Source: CAD feature listing. Evaluate the final solid. Frame: model axes, mm. Face numbers are marked on the shaded views. A direction names the side the tool comes from. Coordinates: 2 decimals unless noted, no trailing zeros. Write each loop counter-clockwise with the first axis right and the second up, starting at its lowest first coordinate (ties: lowest second). Pieces come first, ordered by that corner, then holes. Notation, with made-up numbers: (11.5, 14.25) -> (18.5, 14.25) arc R16 ccw to (18.5, 38.25) -> close; hole circle Ø7 at (76, 12.25). An arc over 180 degrees is marked (long way). One line per item, written item: value. Start each with the question number.
1. Section query A-A, the plane x = -12.7. State how many separate pieces and enclosed holes the cut face has, and give its area (3 significant figures).
2. First-contact query: P1, Ø4, axis at x = -20.64, y = 38.1, coming from the -Z side; P2, Ø7.5, axis at x = -44.45, y = 38.1, coming from the -Z side; P3, Ø12.5, axis at x = -21.5, z = -4, coming from the +Y side; P4, Ø8, axis at y = 25, z = -43.5, coming from the -X side. Flat tips, straight axial feed; report the tip coordinate or a pass-through.
3. Mould query, pull axis Z, two halves, no side actions, for the marked faces 5, 6 and 7. Classes: released by +Z, released by -Z, zero draft, split by the parting line, or undercut.
4. Section query B-B, the plane y = -24. Output: boundary loops of the cut face in (x, z), and give its area (3 significant figures).
5. Line query: line 1 (Y direction, x = -44.45, z = -15.25) (3 decimals); line 2 (Y direction, x = -12, z = -50); line 3 (Y direction, x = -8.5, z = -30). Output: solid intervals per line, ascending.
6. Access query for the marked faces 1, 2, 3 and 4. Directions: +Z, -Z, +X, -X, +Y, -Y. A direction counts if a zero-diameter tool reaches every point of the face in a straight line with its end or side. Return the directions, or none.
7. Section query D-D, the plane x = 5.5. Output: boundary loops of the cut face in (y, z), and give its area (3 significant figures).
8. Section query C-C, the plane y = 10.5. Output: boundary loops of the cut face in (x, z), and give its area (3 significant figures).
Autodesk Inventor part; units mm, degrees
ref_plane "Work Plane1" through (0, 0, -31.75) normal (0, 0, 1) x (1, 0, 0)
ref_plane "Work Plane2" through (0, 31.75, -63.5) normal (0, -1, 0) x (1, 0, 0)
ref_plane "YZ Plane" through (0, 0, 0) normal (1, 0, 0) x (0, 1, 0)
sketch "Sketch1" plane through (0, 0, 0) normal (0, 0, 1) x (1, 0, 0)
  arc A0 (-50.8, 31.75) -> (-50.8, -31.75) centre (-50.8, 0) ccw
  line L0 (-50.8, 31.75) -> (0, 31.75)
  line L1 (0, -31.75) -> (-50.8, -31.75)
  arc A1 (0, -31.75) -> (0, 31.75) centre (0, 0) ccw
extrude "Extrusion1" add sketch "Sketch1" against normal blind 63.5
ref_plane "Work Plane1" through (0, 0, -31.75) normal (0, 0, 1) x (1, 0, 0)
sketch "Sketch2" plane through (0, 0, -31.75) normal (0, 0, 1) x (1, 0, 0)
  arc A0 (-50.8, 31.75) -> (-50.8, -31.75) centre (-50.8, 0) ccw
  line L0 (-50.8, 31.75) -> (0, 31.75)
  arc A1 (0, -31.75) -> (0, 31.75) centre (0, 0) ccw
  line L1 (0, -31.75) -> (-50.8, -31.75)
  arc A2 (-50.8, 28.1437) -> (-50.8, -28.1437) centre (-50.8, 0) ccw
  line L2 (-50.8, 28.1437) -> (0, 28.1437)
  arc A3 (0, -28.1437) -> (0, 28.1437) centre (0, 0) ccw
  line L3 (0, -28.1437) -> (-50.8, -28.1437)
extrude "Extrusion2" cut sketch "Sketch2" along normal mid plane 55.88 contours L2 A3 L3 A2
sketch "Sketch3" plane through (0, 0, 0) normal (0, 0, 1) x (1, 0, 0)
  circle A0 centre (0, 0) radius 31.75
  line L0 (0, 31.75) -> (19.0425, -25.4056)
  dimension "d7" = 63.5
extrude "Extrusion3" cut sketch "Sketch3" against normal blind 63.5 contours A0 L0 picked at (8.7025, 12.4328)
sketch "Sketch4" plane through (-50.8, 31.75, 0) normal (0, 1, 0) x (1, 0, 0)
  line L0 (50.8, 0) -> (0, 0)
  line L1 (50.8, 0) -> (50.8, 63.5)
  line L2 (0, 63.5) -> (50.8, 63.5)
  line L3 (0, 0) -> (0, 63.5)
  line L4 (0, 31.75) -> (50.8, 31.75)
  line L5 (0, 0) -> (0, 63.5)
  line L6 (50.8, 0) -> (50.8, 63.5)
  line L7 (0, 11.43) -> (50.8, 11.43)
  line L8 (50.8, 11.43) -> (50.8, 52.07)
  line L9 (50.8, 52.07) -> (0, 52.07)
  line L10 (0, 52.07) -> (0, 11.43)
  line L11 (0, 19.3675) -> (50.8, 19.3675)
  line L12 (0, 44.1325) -> (50.8, 44.1325)
  dimension "d10" = 31.75
  dimension "d11" = 20.32
  dimension "d12" = 40.64
  dimension "d13" = 7.9375
  dimension "d14" = 7.9375
extrude "Extrusion4" add sketch "Sketch4" along normal blind 12.7 contours L7 L3 L11 L1 | L12 L3 L9 L1
sketch "Sketch5" plane through (-50.8, 31.75, -11.43) normal (0, 0, 1) x (1, 0, 0)
  line L0 (50.8, 0) -> (0, 0)
  line L1 (50.8, 0) -> (50.8, 12.7)
  line L2 (0, 12.7) -> (50.8, 12.7)
  line L3 (0, 0) -> (0, 12.7)
  circle A0 centre (6.35, 6.35) radius 6.35
  circle A1 centre (44.45, 6.35) radius 6.35
  line L4 (6.35, 12.7) -> (44.45, 12.7)
  line L5 (44.45, 0) -> (6.35, 0)
  line L6 (6.35, 6.35) -> (0, 6.35)
  line L7 (44.45, 6.35) -> (50.8, 6.35)
  point P0 (50.8, -31.75)
extrude "Extrusion5" cut sketch "Sketch5" against normal blind 63.5 contours A1 L2 L1 | L3 L2 A0
sketch "Sketch6" plane through (-50.8, 31.75, -11.43) normal (0, 0, 1) x (1, 0, 0)
  arc A0 (6.35, 12.7) -> (0, 6.35) centre (6.35, 6.35) ccw
  line L0 (0, 0) -> (0, 6.35)
  line L1 (50.8, 0) -> (0, 0)
  line L2 (50.8, 0) -> (50.8, 6.35)
  arc A1 (50.8, 6.35) -> (44.45, 12.7) centre (44.45, 6.35) ccw
  line L3 (6.35, 12.7) -> (44.45, 12.7)
  circle A2 centre (6.35, 6.35) radius 3.175
  line L4 (6.35, 6.35) -> (44.45, 6.35)
  circle A3 centre (14.2875, 6.35) radius 3.175
  circle A4 centre (22.225, 6.35) radius 3.175
  circle A5 centre (30.1625, 6.35) radius 3.175
  circle A6 centre (38.1, 6.35) radius 3.175
  point P0 (50.8, -31.75)
  dimension "d22" = 7.9375
  dimension "d31" = 6.35
extrude "Extrusion6" cut sketch "Sketch6" against normal blind 63.5 contours A2 | A6 L4 | L4 A6 | A5 L4 | L4 A5 | A4 L4 | L4 A4 | A3 L4 | L4 A3
ref_plane "Work Plane2" through (0, 31.75, -63.5) normal (0, -1, 0) x (1, 0, 0)
sketch "Sketch8" plane through (0, 31.75, -63.5) normal (0, -1, 0) x (1, 0, 0)
  line L0 (-50.8, 63.5) -> (-50.8, 63.5)
  line L1 (-50.8, 63.5) -> (-50.8, 52.07)
  line L2 (-50.8, 52.07) -> (-50.8, 44.1325)
  line L3 (-50.8, 44.1325) -> (-50.8, 19.3675)
  line L4 (-50.8, 19.3675) -> (-50.8, 11.43)
  line L5 (-50.8, 11.43) -> (-50.8, 0)
  line L6 (-50.8, 0) -> (-50.8, 0)
  line L7 (-50.8, 63.5) -> (-50.8, 0)
  line L8 (-50.8, 63.5) -> (-82.55, 63.5)
  line L9 (-82.55, 63.5) -> (-82.55, 0)
  line L10 (-82.55, 0) -> (-50.8, 0)
  line L11 (-50.8, 59.69) -> (-78.9437, 59.69)
  line L12 (-54.4877, 59.69) -> (-50.8, 59.69)
  line L13 (-78.9437, 3.81) -> (-78.9437, 59.69)
  line L14 (-50.8, 59.69) -> (-82.55, 59.69)
  line L15 (-78.9437, 59.69) -> (-78.9437, 3.81)
  line L16 (-82.55, 3.81) -> (-50.8, 3.81)
  line L17 (-50.8, 3.81) -> (-50.8, 59.69)
  line L18 (-82.55, 59.69) -> (-82.55, 3.81)
  line L19 (-50.8, 63.5) -> (-82.55, 63.5)
  line L20 (-82.55, 63.5) -> (-82.55, 59.69)
  line L21 (-82.55, 59.69) -> (-50.8, 59.69)
  line L22 (-50.8, 59.69) -> (-50.8, 63.5)
  line L23 (-78.9437, 59.69) -> (-50.8, 59.69)
  line L24 (-50.8, 59.69) -> (-50.8, 3.81)
  line L25 (-50.8, 3.81) -> (-78.9437, 3.81)
  line L26 (-78.9437, 3.81) -> (-78.9437, 59.69)
  line L27 (-82.55, 3.81) -> (-50.8, 3.81)
  line L28 (-50.8, 3.81) -> (-50.8, 0)
  line L29 (-50.8, 0) -> (-82.55, 0)
  line L30 (-82.55, 0) -> (-82.55, 3.81)
  point P0 (0, 63.5)
extrude "Extrusion7" cut sketch "Sketch8" along normal blind 31.75 contours L1 L2 L3 L4 L5 L16 L13 L11 | L14 L13 L16 L9
properties part number "Scoop_001"
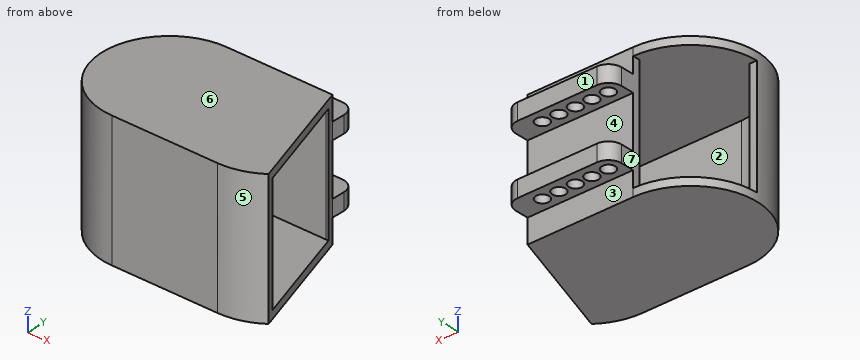
Computed values:
1. separate pieces: 3
1. enclosed holes: 1
1. area: 988 mm²
2. P1: passes through
2. P2: stops at z = -52.07
2. P3: stops at y = 31.75
2. P4: stops at x = -50.8
3. face 5: zero draft
3. face 6: released by +Z
3. face 7: undercut
4. outline: (-71.59, -63.5) -> (18.57, -63.5) -> (18.57, 0) -> (-71.59, 0) -> close; hole (-65.5, -59.69) -> (14.7, -59.69) -> (14.7, -3.81) -> (-65.5, -3.81) -> close
4. area: 1,240 mm²
5. line 1: y = -31.75 to -28.144, 28.144 to 34.925, 41.275 to 44.45
5. line 2: y = -31.75 to -28.14, 28.14 to 35, 41.2 to 44.45
5. line 3: y = -31.75 to -28.14, 28.14 to 31.75
6. face 1: +Z, -Z, +X, -X, +Y
6. face 2: none
6. face 3: -Z, +X, -X, +Y
6. face 4: +X, -X, +Y
7. outline: (-31.27, -63.5) -> (15.24, -63.5) -> (15.24, -59.69) -> (-27.6, -59.69) -> (-27.6, -3.81) -> (15.24, -3.81) -> (15.24, 0) -> (-31.27, 0) -> close
7. area: 559 mm²
8. outline: (-80.76, -63.5) -> (7.08, -63.5) -> (7.08, -59.69) -> (-80.76, -59.69) -> close; (-80.76, -3.81) -> (7.08, -3.81) -> (7.08, 0) -> (-80.76, 0) -> close
8. area: 669 mm²
